Design review of the part shown in the three views and the two pictorial views. Dimensions are in mm from the part's minimum x, y and z. A direction names the side the tool comes from. Round coordinates to 2 decimals unless told otherwise and drop trailing zeros. Order: outer loops, then holes, each group sorted by start corner. A loop starts at its lowest first (then second) coordinate and runs counter-clockwise, first axis right, second up. Notation, with made-up numbers: (-11, -32) - (37, -32) arc R9 cw to (37, -26) - close; hole circle Ø7 at (67, -10). An arc over 180 degrees is marked (long way). One line per item, written item: value.
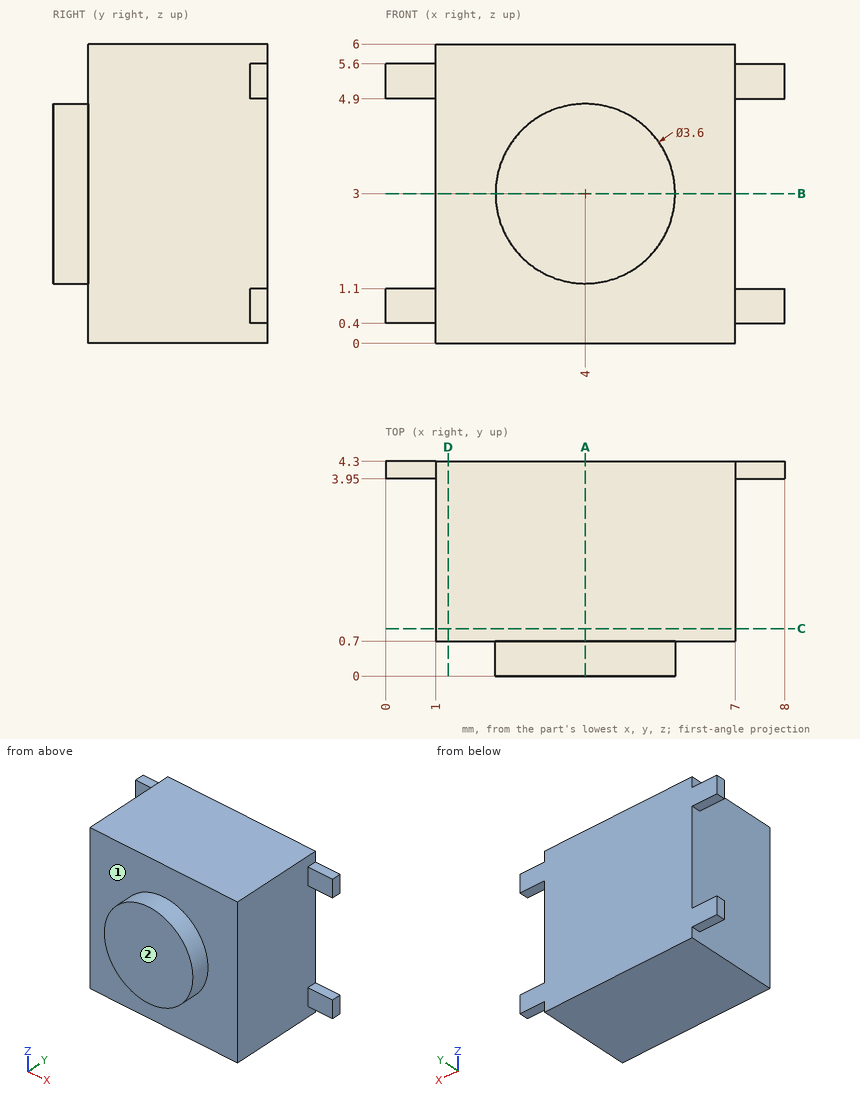
Item 1: Take a section at A-A (x = 4). Write out the cut boundary in (y, z), plus the area to 3 significant figures.
Returned:
outline: (0, 1.2) - (0.7, 1.2) - (0.7, 0) - (4.3, 0) - (4.3, 6) - (0.7, 6) - (0.7, 4.8) - (0, 4.8) - close
area: 24.1 mm^2
Item 2: Wall thickness on line 1 (Y direction, x = 6.25, z = 2.85); line 2 (X direction, y = 2.65, z = 1.65); line 3 (X direction, y = 0.2, z = 1.45): over which ranges is each line inside the solid? List them lowest first.
Returned:
line 1: 0.7 to 4.3
line 2: 1 to 7
line 3: 3.08 to 4.92
Item 3: Take a section at B-B (z = 3). Write out the cut boundary in (x, y).
Returned:
outline: (1, 0.7) - (2.2, 0.7) - (2.2, 0) - (5.8, 0) - (5.8, 0.7) - (7, 0.7) - (7, 4.3) - (1, 4.3) - close
Item 4: Machinability: for the marked faces 1 and 2, which of the approach directions +Z, -Z, +X, -X, +Y, -Y give a long, thin tool a straight path to every point of the face, cutting with its end or side? Answer none if there is none.
Returned:
face 1: -Y
face 2: +Z, -Z, +X, -X, -Y
Item 5: Take a section at D-D (x = 1.25). Write out the cut boundary in (y, z), plus the area to 3 significant figures.
Returned:
outline: (0.7, 0) - (4.3, 0) - (4.3, 6) - (0.7, 6) - close
area: 21.6 mm^2
Item 6: Take a section at C-C (y = 0.95). Write out the cut boundary in (x, z).
Returned:
outline: (1, 0) - (7, 0) - (7, 6) - (1, 6) - close
Item 7: For P1, Ø0.8, axis at x = 7.5, z = 5, coming from the -Y side; P2, Ø1, axis at y = 1.5, z = 2, coming from the +X side; P3, Ø1.8, axis at y = 1.5, z = 2.5, coming from the -X side, all flat-tipped, find the tip position at first contact; note any pin that passes through.
Returned:
P1: y = 3.95
P2: x = 7
P3: x = 1
